For this review, take the finished solid that the model builds, in its own axes (mm). Give positions to 0.01 mm unless a question says otherwise; leave off trailing zeros. Loops run counter-clockwise (first coordinate to the right, second up) from the corner with the lowest first, then second, coordinate; pieces in that order, holes last. Notation, with made-up numbers: (24, 55) - (41, 55) arc R6 ccw to (41, 59) - close; hole circle Ø5 at (-19.75, -10). An arc over 180 degrees is marked (long way). Put each result on its own line as item: value.
from build123d import *

# Parameters (mm, degrees)
SKETCH1_W           = 482.6
SKETCH1_H           = 50.8
BOSS_EXTRUDE1_DEPTH = 3.175
SKETCH2_R           = 12.7
CUT_EXTRUDE1_DEPTH  = 486.276705216
LPATTERN1_COUNT     = 15
LPATTERN1_PITCH     = 36.068


with BuildPart() as part:
    # Sketch1 → Boss-Extrude1 (new body)
    with BuildSketch(Plane.XY):
        with Locations((241.3, 25.4)):
            Rectangle(SKETCH1_W, SKETCH1_H)
    extrude(amount=BOSS_EXTRUDE1_DEPTH)

    # Sketch2 → Cut-Extrude1 (cut, through all)
    with BuildSketch(Plane.XY.offset(3.175)):
        with Locations((25.4, 25.4)):
            Circle(SKETCH2_R)
    cut_extrude1 = extrude(amount=-CUT_EXTRUDE1_DEPTH, mode=Mode.SUBTRACT)

    # LPattern1: Cut-Extrude1 ×15
    with Locations(*[(i * LPATTERN1_PITCH, 0, 0) for i in range(1, LPATTERN1_COUNT)]):
        add(cut_extrude1, mode=Mode.SUBTRACT)


solid = part.part
1) Wall thickness on line 1 (Y direction, x = 25.4, z = 2.35); line 2 (Y direction, x = 355, z = 3.05): over which ranges is each line inside the solid? List them lowest first.
Geometry check:
line 1: y = 0 to 12.7, 38.1 to 50.8
line 2: y = 0 to 13.72, 37.08 to 50.8
2) Draft analysis for pull direction X (two halves, no side actions). For faces 1 (the face through (412.788, 33.983, 1.61)), 2 (the face through (176.5, 36.11, 1.61)), 3 (the face through (238, 43, 0)), state which applies: pulls with the +X half, pulls with the -X half, needs draft (parallel to the pull), parting line crosses it, or undercut.
Geometry check:
face 1: undercut
face 2: undercut
face 3: needs draft
3) Take a section at B-B on y = 25.4. State how many separate pieces and enclosed holes the cut face has, and give its area (3 significant figures).
Geometry check:
separate pieces: 14
enclosed holes: 0
area: 481 mm²
4) Take a section at A-A on x = 386.08. State the section outline as (y, z) points (3 decimals).
Geometry check:
outline: (0, 0) - (12.7, 0) - (12.7, 3.175) - (0, 3.175) - close; (38.1, 0) - (50.8, 0) - (50.8, 3.175) - (38.1, 3.175) - close
